The model under review builds one solid part; all positions refer to its coordinate system, in mm. A direction names the side the tool comes from. Round coordinates to 2 decimals unless told otherwise and drop trailing zeros. Order: outer loops, then holes, each group sorted by start corner. A loop starts at its lowest first (then second) coordinate and runs counter-clockwise, first axis right, second up. Notation, with made-up numbers: M 36,33 L 88,33 A20 cw 88,61 Z; hole C 88,-38 d5. An arc over 180 degrees is marked long. Answer as a JSON object with one key per item and string values. Group by question number.
1. Add section D-D on x = 74.93. State the section outline as (y, z) points (3 decimals), and give its area (3 significant figures).
2. Machinability: for faces 1 (the face through (1, 69.85, 3)), 2 (the face through (-81.28, 62, 3)), 3 (the face through (-1, 79.375, 3)), 4 (the face through (81.28, 62, 3)), which of the approach directions +Z, -Z, +X, -X, +Y, -Y give a long, thin tool a straight path to every point of the face, cutting with its end or side? Answer none if there is none.
3. Add section A-A on y = 24.13. State the section outline as (x, z) points, and give its area (3 significant figures).
4. To check wall thickness, follow probe 1 along Y at (x, z) = (-74.93, 1.5) (3 decimals); probe 2 along X at (y, z) = (-24, 2); probe 3 along Y at (x, z) = (14.5, 3.75) (3 decimals). State the ranges of each line that lie inside material, in increasing order. Write a range as [from, to].
5. Clearance check with flat-ended pins moving along their axes: P1, Ø1.5, axis at y = 47.5, z = 3.5, coming from the +X side; P2, Ø4.5, axis at x = 74.93, y = -29.21, coming from the -Z side; P3, Ø1.9, axis at y = 64.5, z = 1.5, coming from the -X side; P4, Ø1.9, axis at x = 114, z = 4.5, coming from the +Y side. State where each tip first meets the part, or that it passes through.
6. Mouldability with a two-part tool opening along X and no side actions: class faces 5 (the face through (116.244, 24.878, 3.131)), 6 (the face through (123.19, -1, 3)), 7 (the face through (-2, -38.1, 3)) as released by +X, released by -X, zero draft, split by the parting line, or undercut.
7. Add section B-B on z = 2.5. Give the number of separate pieces and of enclosed holes in the cut face, and give its area (3 significant figures).
8. Add section C-C on x = -5. State the section outline as (y, z) points (3 decimals).
```python
from build123d import *

# Parameters (mm, degrees)
SKETCH1_W              = 246.38
SKETCH1_H              = 76.2
BOSS_EXTRUDE1_DEPTH    = 6.35
F_10_CLEARANCE_HOLE1_D = 4.9784
BOSS_EXTRUDE2_DEPTH    = 6.35
FILLET1_R              = 12.7
FILLET1_OF_MIRROR1_R   = 12.7
FILLET2_R              = 6.35
FILLET3_R              = 6.35


with BuildPart() as part:
    # Sketch1 → Boss-Extrude1 (new body)
    with BuildSketch(Plane.XY):
        Rectangle(SKETCH1_W, SKETCH1_H)
    extrude(amount=BOSS_EXTRUDE1_DEPTH)

    # #10 Clearance Hole1 (through all)
    with Locations(Plane.XY.offset(6.35)):
        with Locations((-74.93, 29.21), (-74.93, -29.21), (74.93, 29.21), (74.93, -29.21), (-118.618, 24.13), (-118.618, -24.13), (118.618, 24.13), (118.618, -24.13)):
            Hole(F_10_CLEARANCE_HOLE1_D / 2)

    # Sketch5 → Boss-Extrude2 (add)
    with BuildSketch(Plane.XY.offset(6.35)):
        Polygon((-81.28, 47.271427301), (-81.28, 38.1), (-68.58, 38.1), (-68.58, 69.85), (-81.28, 69.85), align=None)
        Polygon((-81.28, 69.85), (-68.58, 69.85), (0, 69.85), (0, 79.375), (-81.28, 79.375), align=None)
    boss_extrude2 = extrude(amount=-BOSS_EXTRUDE2_DEPTH)

    # Fillet1
    fillet1_edges = [part.edges().sort_by_distance(p)[0] for p in [
        (-68.58, 69.85, 3.175),
    ]]
    fillet(fillet1_edges, radius=FILLET1_R)

    # Mirror1: Boss-Extrude2 across plane
    add(boss_extrude2.mirror(Plane(origin=(0, 0, 0), x_dir=(0, 0, 1), z_dir=(1, 0, 0))))

    # Fillet1 of Mirror1
    fillet1_of_mirror1_edges = [part.edges().sort_by_distance(p)[0] for p in [
        (68.58, 69.85, 3.175),
    ]]
    fillet(fillet1_of_mirror1_edges, radius=FILLET1_OF_MIRROR1_R)

    # Fillet2
    fillet2_edges = [part.edges().sort_by_distance(p)[0] for p in [
        (68.58, 38.1, 3.175),
        (-68.58, 38.1, 3.175),
    ]]
    fillet(fillet2_edges, radius=FILLET2_R)

    # Fillet3
    fillet3_edges = [part.edges().sort_by_distance(p)[0] for p in [
        (81.28, 38.1, 3.175),
        (-81.28, 38.1, 3.175),
    ]]
    fillet(fillet3_edges, radius=FILLET3_R)


solid = part.part
```
Recorded:
{
 "1": {"outline": "M -38.1,0 L -31.699,0 L -31.699,6.35 L -38.1,6.35 Z; M -26.721,0 L 26.721,0 L 26.721,6.35 L -26.721,6.35 Z; M 31.699,0 L 79.375,0 L 79.375,6.35 L 31.699,6.35 Z", "area": "683 mm²"},
 "2": {"face 1": "+Z, -Z", "face 2": "+Z, -Z, -X, +Y", "face 3": "+Z, -Z, +X, -X, +Y", "face 4": "+Z, -Z, +X, +Y"},
 "3": {"outline": "M -123.19,0 L -121.11,0 L -121.11,6.35 L -123.19,6.35 Z; M -116.13,0 L 116.13,0 L 116.13,6.35 L -116.13,6.35 Z; M 121.11,0 L 123.19,0 L 123.19,6.35 L 121.11,6.35 Z", "area": "1,500 mm²"},
 "4": {"probe 1": "y = [-38.1, -31.699], [-26.721, 26.721], [31.699, 79.375]", "probe 2": "x = [-123.19, -121.1], [-116.13, 116.13], [121.1, 123.19]", "probe 3": "y = [-38.1, 38.1], [69.85, 79.375]"},
 "5": {"P1": "stops at x = 81.28", "P2": "passes through", "P3": "stops at x = -81.28", "P4": "stops at y = 38.1"},
 "6": {"face 5": "undercut", "face 6": "released by +X", "face 7": "zero draft"},
 "7": {"separate pieces": "1", "enclosed holes": "9", "area": "21,100 mm²"},
 "8": {"outline": "M -38.1,0 L 38.1,0 L 38.1,6.35 L -38.1,6.35 Z; M 69.85,0 L 79.375,0 L 79.375,6.35 L 69.85,6.35 Z"}
}
